Input: part model. Units: mm. Frame: model coordinates. Give positions to 0.01 mm unless a question says otherwise; leave off trailing zeros. Loops run counter-clockwise (first coordinate to the right, second up) from the corner with the lowest first, then second, coordinate; pieces in that order, holes last. Notation, with made-up numbers: M -27,0.25 L -18,0.25 A17 ccw -18,27.25 Z; hole C 43,87.5 d5. An arc over 180 degrees is marked long. Return JSON: item names as keys, results as strings. Group by question number.
```python
from build123d import *

# Parameters (mm, degrees)
F4_R     = 3.175
F5_DEPTH = 6.35
F7_R     = 3.175
F8_DEPTH = 9.525


with BuildPart() as f2:
    # F0 (on Front) → F2 (revolve)
    with BuildSketch(Plane.XZ):
        with BuildLine():
            Line((0, -12.7), (0, 12.7))
            ThreePointArc((0, 12.7), (-12.7, 0), (0, -12.7))
        make_face()
    revolve(axis=Axis((0, 0, 0), (0, 0, 1)))

    # F4 (on offset) → F5 (cut)
    with BuildSketch(Plane.XZ.offset(12.7)):
        Circle(F4_R)
    extrude(amount=-F5_DEPTH, mode=Mode.SUBTRACT)


with BuildPart() as f8:
    # F7 (on offset) → F8 (new body)
    with BuildSketch(Plane.XZ.offset(-12.7)):
        Circle(F7_R)
    extrude(amount=F8_DEPTH)


solid = f2.part
```
Item 1: First-contact query: pin 1 Ø12 at (y, z) = (-6.5, -1) entering from -X; pin 2 Ø10 at (x, z) = (3.5, -2.5) entering from -Y; pin 3 Ø1 at (x, y) = (4.5, -2) entering from +Z; pin 4 Ø6 at (x, y) = (1.5, 2) entering from +Z. Flat tips, straight axial feed; report the tip coordinate or a pass-through.
Item 2: Section B-B, the plane z = -10. Return loops of the section in (x, y), then the cut area to 3 significant figures.
Item 3: Section D-D, the plane y = -8.25. Return loops of the section in (x, z) (3 decimals), then the cut area to 3 significant figures.
Item 4: Material intervals for line 1 (Z direction, x = 0, y = -9.5) (3 decimals); line 2 (Z direction, x = 0, y = -10.6) (3 decimals); line 3 (X direction, y = -10.1, z = 0) (3 decimals), sorted ascending. Write a range as from..to.
Item 5: Section C-C, the plane y = 10.5. Return loops of the section in (x, z), then the cut area to 3 significant figures.
Item 6: Section A-A, the plane x = 0. Return loops of the section in (y, z) (3 decimals), then the cut area to 3 significant figures.
Answer below:
{
 "1": {"pin 1": "x = -12.69", "pin 2": "y = -12.3", "pin 3": "z = 11.9", "pin 4": "z = 12.7"},
 "2": {"outline": "C 0,0 d15.66", "area": "193 mm^2"},
 "3": {"outline": "C 0,0 d19.311; hole C 0,0 d6.35", "area": "261 mm^2"},
 "4": {"line 1": "-8.429..-3.175, 3.175..8.429", "line 2": "-6.995..-3.175, 3.175..6.995", "line 3": "-7.699..-3.175, 3.175..7.699"},
 "5": {"outline": "C 0,0 d14.29", "area": "160 mm^2"},
 "6": {"outline": "M -12.297,-3.175 A12.7 ccw long -12.297,3.175 L -6.35,3.175 L -6.35,-3.175 Z", "area": "467 mm^2"}
}
